The listing builds one solid part. Answer for the finished solid, in the listing's coordinates (mm). A direction names the side the tool comes from. Give positions to 0.01 mm unless a question says otherwise; leave off trailing zeros. Write each loop counter-clockwise with the first axis right and the second up, starting at its lowest first coordinate (ties: lowest second). Pieces come first, ordered by that corner, then holes. Notation, with made-up numbers: M 42.25,50.5 L 85.25,50.5 A26 cw 85.25,79.5 Z; hole C 77.25,84 d10. An arc over 180 degrees is marked long. Answer as a JSON object with one key per item and string values.
```python
from build123d import *

# Parameters (mm, degrees)
BOSS_EXTRUDE1_DEPTH = 38.1
BOSS_EXTRUDE2_DEPTH = 19.05
BOSS_EXTRUDE3_DEPTH = 19.05


with BuildPart() as part:
    # Sketch2 → Boss-Extrude1 (new body)
    with BuildSketch(Plane.XY):
        with BuildLine():
            Line((0, 159.7945402), (24.767030522, 124.423554927))
            Line((24.767030522, 124.423554927), (235.653251342, 272.08767645))
            ThreePointArc((235.653251342, 272.08767645), (282.133094114, 178.538387025), (240.963304039, 82.533732339))
            ThreePointArc((240.963304039, 82.533732339), (209.988023007, 44.978276319), (191.364517126, 0))
            ThreePointArc((191.364517126, 0), (89.764517126, -79.406163555), (-11.835482874, 0))
            ThreePointArc((-11.835482874, 0), (-30.458988755, 44.978276319), (-61.434269787, 82.533732339))
            ThreePointArc((-61.434269787, 82.533732339), (-76.883813046, 250.879864381), (89.764517126, 279.295399058))
            ThreePointArc((89.764517126, 279.295399058), (100.369013371, 285.48693454), (111.532091006, 290.603197817))
            Line((111.532091006, 290.603197817), (-24.767030522, 195.165525472))
            Line((-24.767030522, 195.165525472), (0, 159.7945402))
        make_face()
    extrude(amount=BOSS_EXTRUDE1_DEPTH)



with BuildPart() as body_2:
    # Sketch3 → Boss-Extrude2 (new body)
    with BuildSketch(Plane(origin=(0, 0, 0), x_dir=(-1, 0, 0), z_dir=(0, 0, -1))):
        with BuildLine():
            Line((24.767030522, 195.165525472), (-24.767030522, 124.423554927))
            Line((-24.767030522, 124.423554927), (-235.653251342, 272.08767645))
            ThreePointArc((-235.653251342, 272.08767645), (-176.097486655, 298.136787359), (-111.532091006, 290.603197817))
            Line((-111.532091006, 290.603197817), (24.767030522, 195.165525472))
        make_face()
    extrude(amount=-BOSS_EXTRUDE2_DEPTH)


with BuildPart() as part_1:
    add(part.part)

    add(body_2.part)  # Boss-Extrude3 merges body 2
    # Sketch4 → Boss-Extrude3 (add)
    with BuildSketch(Plane(origin=(0, 0, 0), x_dir=(-1, 0, 0), z_dir=(0, 0, -1))):
        Polygon((-152.689068197, 231.824942879), (-215.108453971, 275.531467329), (-182.328560634, 322.34600666), (-119.909174859, 278.63948221), align=None)
    extrude(amount=-BOSS_EXTRUDE3_DEPTH)


solid = part_1.part
```
1. For faces 4 (the cylindrical face through (-78.45, 248.8, 18.78)), 5 (the flat face through (104, 225, 19.05)), determine the directions among +Z, -Z, +X, -X, +Y, -Y from which every point of the face is accessible in a straight line to the end or side of a thin tool.
Verdict:
{"face 4": "+Z, -Z", "face 5": "+Z"}
2. The mould has two halves that part along Y. Classify faces 1 (the flat face through (44.337, 243.552, 28.442)), 2 (the flat face through (87, 124, 0)), 3 (the cylindrical face through (-30.108, 44.391, 18.783)): released by +Y, released by -Y, zero draft, split by the parting line, or undercut.
Verdict:
{"face 1": "undercut", "face 2": "zero draft", "face 3": "released by -Y"}
3. A cutting plane is placed at B-B, the plane y = 220.5. Give the vertices of the cut face in (x, z).
Verdict:
{"outline": "M -94.06,0 L 273.59,0 L 273.59,38.1 L 161.98,38.1 L 161.98,19.05 L 11.41,19.05 L 11.41,38.1 L -94.06,38.1 Z"}
4. A cutting plane is placed at C-C, the plane x = 73.5. Give the vertices of the cut face in (y, z).
Verdict:
{"outline": "M -78.14,0 L 288.25,0 L 288.25,38.1 L 263.97,38.1 L 263.97,19.05 L 158.55,19.05 L 158.55,38.1 L -78.14,38.1 Z"}
5. Consider line 1 along Z through (x, y) = (87, 171); line 2 along Y through (x, z) = (69, 32); line 3 along Y through (x, z) = (147.5, 3.5). Determine where each line is inside the solid, lowest interval first.
Verdict:
{"line 1": "z = 0 to 19.05", "line 2": "y = -77.33 to 155.4, 260.82 to 290.2", "line 3": "y = -62.05 to 299.08"}
6. A cutting plane is placed at A-A, the plane z = 33.5. Give the vertices of the cut face in (x, y).
Verdict:
{"outline": "M -61.43,82.53 A164.45 cw -11.84,0 A104.7 ccw 191.36,0 A164.45 cw 240.96,82.53 A124.45 ccw 235.65,272.09 L 24.77,124.42 L -24.77,195.17 L 111.53,290.6 A124.45 ccw 89.76,279.3 A124.45 ccw Z"}
7. A cutting plane is placed at D-D, the plane x = 158. Give the vertices of the cut face in (y, z), plus the area to 3 significant figures.
Verdict:
{"outline": "M -54.12,0 L 305.31,0 L 305.31,19.05 L 217.71,19.05 L 217.71,38.1 L -54.12,38.1 Z", "area": "12,000 mm2"}
8. Flat-ended cylindrical pins translate along their axes: pin 1 (2 mm diameter, centred on x = 211, z = 17, fed in from +Y); pin 2 (8 mm diameter, centred on x = 154, y = 246, fed in from +Z); pin 3 (1 mm diameter, centred on y = 170, z = 33.5, fed in from +X); pin 4 (5 mm diameter, centred on x = 95, y = 113.5, fed in from -Z). Find the tip coordinate at first contact, or state that the pin passes through.
Verdict:
{"pin 1": "stops at y = 287.99", "pin 2": "stops at z = 19.05", "pin 3": "stops at x = 282.1", "pin 4": "stops at z = 0"}
